Autodesk Inventor part; units mm, degrees
ref_plane "YZ Plane" through (0, 0, 0) normal (1, 0, 0) x (0, 1, 0)
ref_plane "XZ Plane" through (0, 0, 0) normal (0, 1, 0) x (-1, 0, 0)
ref_plane "XY Plane" through (0, 0, 0) normal (0, 0, 1) x (1, 0, 0)
sketch "Sketch1" plane through (0, 0, 0) normal (0, 1, 0) x (-1, 0, 0)
  line L0 (-24.5, 52) -> (24.5, 52)
  line L1 (24.5, 52) -> (24.5, -52)
  line L2 (24.5, -52) -> (-24.5, -52)
  line L3 (-24.5, -52) -> (-24.5, 52)
  point P0 (0, 0)
  point P1 (0, -52)
  point P2 (24.5, 0)
  dimension "d0" = 104
  dimension "d1" = 49
extrude "Extrusion1" add sketch "Sketch1" along normal blind 5
sketch "Sketch2" plane through (0, 0, 0) normal (0, -1, 0) x (1, 0, 0)
  line L0 (24.5, 46.65) -> (19.15, 46.65)
  line L1 (19.15, 46.65) -> (19.15, 52)
  line L2 (19.15, 52) -> (24.5, 52)
  line L3 (24.5, 52) -> (24.5, 46.65)
  line L4 (24.5, -52) -> (24.5, 52)
  line L5 (24.5, 52) -> (-24.5, 52)
  line L6 (0, -77) -> (0, 77)
  line L7 (-38.5, 0) -> (38.5, 0)
  line L8 (24.5, -46.65) -> (19.15, -46.65)
  line L9 (19.15, -46.65) -> (19.15, -52)
  line L10 (19.15, -52) -> (24.5, -52)
  line L11 (24.5, -52) -> (24.5, -46.65)
  line L12 (-24.5, 46.65) -> (-19.15, 46.65)
  line L13 (-19.15, 46.65) -> (-19.15, 52)
  line L14 (-19.15, 52) -> (-24.5, 52)
  line L15 (-24.5, 52) -> (-24.5, 46.65)
  line L16 (-19.15, -46.65) -> (-19.15, -52)
  line L17 (-24.5, -46.65) -> (-19.15, -46.65)
  line L18 (-24.5, -52) -> (-24.5, -46.65)
  line L19 (-19.15, -52) -> (-24.5, -52)
  point P0 (0, 0)
  dimension "d4" = 5.35
extrude "Extrusion2" cut sketch "Sketch2" against normal blind 3.35 contours L0 L1 L2 L3 | L4 L10 L9 L8 | L13 L12 L15 L5 | L16 L19 L18 L17
sketch "Sketch3" plane through (0, 5, 0) normal (0, 1, 0) x (1, 0, 0)
  line L0 (-5, -10) -> (-15, -5)
  line L1 (-15, -5) -> (-15, 5)
  line L2 (-15, 5) -> (-5, 10)
  line L3 (-5, 10) -> (-5, -10)
  line L4 (15, -5) -> (15, 5)
  line L5 (15, 5) -> (5, 10)
  line L6 (5, 10) -> (5, -10)
  line L7 (5, -10) -> (15, -5)
  point P0 (0, 0)
  point P1 (-5, 0)
  dimension "d7" = 5
  dimension "d8" = 5
  dimension "d9" = 10
  dimension "d10" = 20
  dimension "d11" = 10
  dimension "d12" = 10
extrude "Extrusion3" cut sketch "Sketch3" against normal through all
chamfer "Chamfer1" distance 2.5 angle 45 8 edges at (5, 0, 0) (-5, 0, 0) (-10, 5, 7.5) (-15, 5, 0) (-10, 5, -7.5) (10, 5, -7.5) (15, 5, 0) (10, 5, 7.5)
equation "\"d4\" = magnet_A"
equation "\"d5\" = magnet_B"
properties part number "BODY_TOP_COVER"
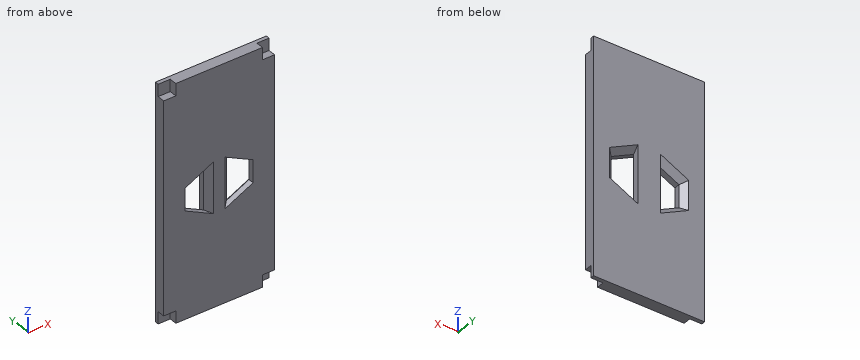
Design review of the part built by this model. Coordinates are the model's own, in mm. Round coordinates to 2 decimals unless told otherwise and drop trailing zeros. Write each loop counter-clockwise with the first axis right and the second up, starting at its lowest first coordinate (ties: lowest second). Pieces come first, ordered by that corner, then holes. Notation, with made-up numbers: (82.5, 1.25) - (109.5, 1.25) arc R11 ccw to (109.5, 15.25) - close; hole circle Ø1 at (57, 49). An arc over 180 degrees is marked (long way). Return JSON: item names as keys, results as strings. Group by question number.
Item 1: For probe 1 along X at (y, z) = (4.55, 12); probe 2 along Z at (x, y) = (-9, 3.15); probe 3 along Z at (x, y) = (-9.5, 3.3), list the stretches that pass through material, from the lowest coordinate up. Write a range as [from, to].
Item 2: We need section D-D on x = -7.5. Write out the cut boundary in (y, z), and give its area (3 significant figures).
Item 3: We need section C-C on y = 1.35. Write out the cut boundary in (x, z).
Item 4: We need section A-A on z = -3. Write out the cut boundary in (x, y), and give its area (3 significant figures).
Item 5: Insertion check: P1, Ø6, axis at x = -21.5, z = -50, coming from the -Y side; P2, Ø1.6, axis at x = 21, z = -48, coming from the -Y side; P3, Ø1.7, axis at x = 21, y = 1, coming from the -Z side; P4, Ø1.7, axis at y = 2, z = -48, coming from the -X side. Each pin has a flat end and moves straight along its axis. Give the tip position at first contact, or say it passes through.
Item 6: We need section B-B on x = -14. Write out the cut boundary in (y, z).
Model answer:
{
 "1": {"probe 1": "x = [-24.5, -5.58], [-5, 5], [5.58, 24.5]", "probe 2": "z = [-52, -8.73], [8.73, 52]", "probe 3": "z = [-52, -8.64], [8.64, 52]"},
 "2": {"outline": "(0, -52) - (5, -52) - (5, -11.54) - (2.5, -8.75) - (0, -8.75) - close; (0, 8.75) - (2.5, 8.75) - (5, 11.54) - (5, 52) - (0, 52) - close", "area": "426 mm²"},
 "3": {"outline": "(-24.5, -46.65) - (-19.15, -46.65) - (-19.15, -52) - (19.15, -52) - (19.15, -46.65) - (24.5, -46.65) - (24.5, 46.65) - (19.15, 46.65) - (19.15, 52) - (-19.15, 52) - (-19.15, 46.65) - (-24.5, 46.65) - close; hole (-15, -5) - (-3.85, -10.57) - (-3.85, 10.57) - (-15, 5) - close; hole (3.85, -10.57) - (15, -5) - (15, 5) - (3.85, 10.57) - close"},
 "4": {"outline": "(-24.5, 0) - (-15, 0) - (-15, 2.5) - (-17.5, 5) - (-24.5, 5) - close; (-5, 2.5) - (-2.5, 0) - (2.5, 0) - (5, 2.5) - (5, 5) - (-5, 5) - close; (15, 0) - (24.5, 0) - (24.5, 5) - (17.5, 5) - (15, 2.5) - close", "area": "133 mm²"},
 "5": {"P1": "stops at y = 0", "P2": "stops at y = 3.35", "P3": "stops at z = -46.65", "P4": "stops at x = -19.15"},
 "6": {"outline": "(0, -52) - (5, -52) - (5, -8.29) - (2.5, -5.5) - (0, -5.5) - close; (0, 5.5) - (2.5, 5.5) - (5, 8.29) - (5, 52) - (0, 52) - close"}
}
